Can you work these out from the model? Positions are in its coordinate system, mm. Give positions to 0.01 mm unless a question says otherwise; leave off trailing zeros. Order: outer loops, then holes, each group sorted by start corner. A loop starts at its lowest first (then second) coordinate and runs counter-clockwise, first axis right, second up. Notation, with made-up numbers: (1.5, 9.25) - (55.5, 9.25) arc R8 ccw to (55.5, 16.25) - close; hole circle Ø10 at (38.5, 9). An arc over 180 degrees is marked (long way). Answer as a JSON object with one key per item and string values.
Solid Edge part; units mm, degrees
sketch "Sketch1" plane through (0, 0, 0) normal (0, 0, 1) x (1, 0, 0)
  line L0 (34.641, -20) -> (0, 40)
  line L1 (0, 40) -> (-34.641, -20)
  line L2 (-34.641, -20) -> (34.641, -20)
extrude "Protrusion1" add sketch "Sketch1" along normal up to vertex (56.5685 mm away)
sketch "Sketch2" plane through (0, 0, 0) normal (1, 0, 0) x (0, 1, 0)
  line L0 (-20, 0) -> (0, 56.5685)
extrude "Cutout1" cut sketch "Sketch2" along normal mid plane 391.7611 material side at (0, -10.0471, 28.3009)
pattern_circular "Pattern1" count 3 over 360 about axis through (0, 0, 0) along (0, 0, -1) of "Cutout1"
Q1. I'm going to push flat-ended pins straight in: pin 1 Ø4 at (y, z) = (6, 11.5) entering from -X; pin 2 Ø6 at (y, z) = (4.5, 26.5) entering from +X. Where does each tip first touch, or does it pass through?
Recorded:
{"pin 1": "stops at x = -16.35", "pin 2": "stops at x = 11.8"}
Q2. I need wall thicknesses on L1, parallel to Z at x = -22, y = -11; L2, parallel to Y at x = -0.5, z = 15; L3, parallel to X at y = 7.5, z = 44. Which ranges of each line are inside material? Lowest first, please.
Recorded:
{"L1": "z = 0 to 18.24", "L2": "y = -14.7 to 28.53", "L3": "x = -0.8 to 0.8"}
Q3. We'd pull the mould along Z, two halves only. Please class faces 1 (the face through (-0.485, -12.082, 22.395)), 2 (the face through (0, 4, 0)): released by +Z, released by -Z, zero draft, split by the parting line, or undercut.
Recorded:
{"face 1": "released by +Z", "face 2": "released by -Z"}
Q4. If we section it at C-C, the plane z = 37: Please give me the cut outline in (x, y), then the cut area to 3 significant figures.
Recorded:
{"outline": "(-11.98, -6.92) - (11.98, -6.92) - (0, 13.84) - close", "area": "249 mm^2"}
